Geometry: final body of the model. Coordinates: model frame, mm. Face numbers are marked on the shaded views. A direction names the side the tool comes from. Give positions to 0.01 mm unless a question says otherwise; leave off trailing zeros. Order: outer loops, then holes, each group sorted by start corner. A loop starts at its lowest first (then second) coordinate and runs counter-clockwise, first axis right, second up. Notation, with made-up numbers: (16, 37.5) -> (21, 37.5) arc R28 ccw to (21, 62.5) -> close; hole circle Ø3 at (-29.5, 46). An arc over 180 degrees is marked (long way). Answer in a Markdown table with one row per item. Add a question column.
Q1. Cut plane C-C on y = -7.5. Return the cut outline in (x, z), and give its area (3 significant figures).
Q2. Pull-direction query (Y, two-part tool) for the marked faces 1, 2, 3 and 4; classes: +Y half, -Y half, draft (parallel to the pull), parting line (faces both ways), or undercut.
Q3. Cut plane B-B on z = 5.1. Return the cut outline in (x, y), and give its area (3 significant figures).
Q4. Line query: line 1 along Z through (x, y) = (11, 20); line 2 along X through (y, z) = (-11, 4.85); line 3 along Y through (x, z) = (10, 1.75). Output: solid intervals per line, ascending. Write a range as from..to.
Q5. Cut plane A-A on x = -2.5. Return the cut outline in (y, z), and give its area (3 significant figures).
Q6. Set-up query: the marked faces 5, 6 and 7. Return all of +Z, -Z, +X, -X, +Y, -Y with unobstructed straight access to the full face (end or side cutting, diameter ignored); none if empty.
Q7. Cut plane D-D on x = -15.5. Return the cut outline in (y, z).
Q8. Contact query for flat-ended pins moving along their axis: P1, Ø2, axis at x = 14, z = 4, coming from the -Y side; P2, Ø1.8, axis at x = -10, z = 1.5, coming from the +Y side. Output: stop coordinate, or through.
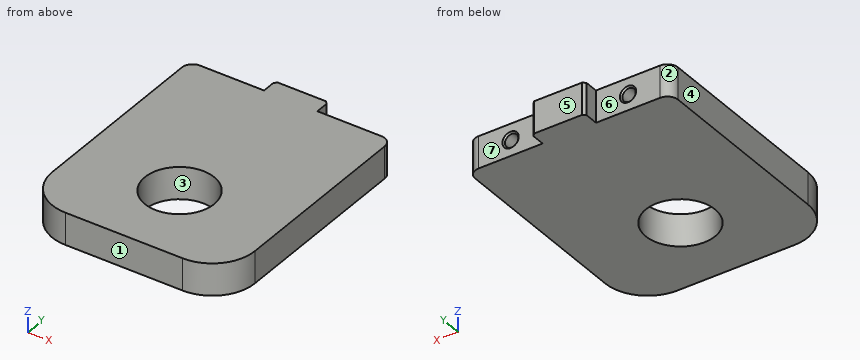
from build123d import *

# Parameters (mm, degrees)
SKETCH_1_W                   = 38
SKETCH_1_H                   = 45
EXTRUDE_1_DEPTH              = 6
SKETCH_2_R                   = 6.5
CUT_EXTRUDE_1_DEPTH          = 31.054117854
FILLET_1_R                   = 2
FILLET_2_R                   = 8
SKETCH_3_W                   = 10
SKETCH_3_H                   = 3
EXTRUDE_2_DEPTH              = 6
CHAMFER_1_SIZE               = 0.5
HOLE_WIZARD_M3_1_D           = 2.5
HOLE_WIZARD_M3_1_DEPTH       = 7.5
HOLE_WIZARD_M3_1_CSINK_D     = 3.05
HOLE_WIZARD_M3_1_CSINK_ANGLE = 90
HOLE_WIZARD_M3_1_TIP         = 0.751075774


with BuildPart() as part:
    # 草图1 → 凸台-拉伸1 (new body)
    with BuildSketch(Plane.XY):
        Rectangle(SKETCH_1_W, SKETCH_1_H)
    extrude(amount=EXTRUDE_1_DEPTH)

    # 草图2 → 切除-拉伸1 (cut, through all)
    with BuildSketch(Plane.XY.offset(6)):
        with Locations((0, -7.5)):
            Circle(SKETCH_2_R)
    extrude(amount=-CUT_EXTRUDE_1_DEPTH, mode=Mode.SUBTRACT)

    # 圆角1
    fillet_1_edges = [part.edges().sort_by_distance(p)[0] for p in [
        (-19, 22.5, 3),
        (19, 22.5, 3),
    ]]
    fillet(fillet_1_edges, radius=FILLET_1_R)

    # 圆角2
    fillet_2_edges = [part.edges().sort_by_distance(p)[0] for p in [
        (19, -22.5, 3),
        (-19, -22.5, 3),
    ]]
    fillet(fillet_2_edges, radius=FILLET_2_R)

    # 草图3 → 凸台-拉伸2 (add)
    with BuildSketch(Plane.XY.offset(6)):
        with Locations((0, 24)):
            Rectangle(SKETCH_3_W, SKETCH_3_H)
    extrude(amount=-EXTRUDE_2_DEPTH)

    # 倒角1
    chamfer_1_edges = [part.edges().sort_by_distance(p)[0] for p in [
        (-5, 25.5, 3),
        (5, 25.5, 3),
    ]]
    chamfer(chamfer_1_edges, length=CHAMFER_1_SIZE)

    # M3 螺纹孔1
    with Locations(Plane(origin=(-11, 22.5, 3), x_dir=(0, 0, 1), z_dir=(0, 1, 0))):
        with Locations((0, 0), (0, 22)):
            CounterSinkHole(HOLE_WIZARD_M3_1_D / 2, HOLE_WIZARD_M3_1_CSINK_D / 2, depth=HOLE_WIZARD_M3_1_DEPTH, counter_sink_angle=HOLE_WIZARD_M3_1_CSINK_ANGLE)
            with Locations((0, 0, -(HOLE_WIZARD_M3_1_DEPTH + HOLE_WIZARD_M3_1_TIP / 2))):  # 118° drill point
                Cone(0, HOLE_WIZARD_M3_1_D / 2, HOLE_WIZARD_M3_1_TIP, mode=Mode.SUBTRACT)


solid = part.part
Completed:
| question | item | result |
|---|---|---|
| 1 | outline | (-19, 0) -> (-6.5, 0) -> (-6.5, 6) -> (-19, 6) -> close; (6.5, 0) -> (19, 0) -> (19, 6) -> (6.5, 6) -> close |
| 1 | area | 150 mm² |
| 2 | face 1 | -Y half |
| 2 | face 2 | +Y half |
| 2 | face 3 | undercut |
| 2 | face 4 | draft |
| 3 | outline | (-19, -14.5) arc R8 ccw to (-11, -22.5) -> (11, -22.5) arc R8 ccw to (19, -14.5) -> (19, 20.5) arc R2 ccw to (17, 22.5) -> (5, 22.5) -> (5, 25) -> (4.5, 25.5) -> (-4.5, 25.5) -> (-5, 25) -> (-5, 22.5) -> (-17, 22.5) arc R2 ccw to (-19, 20.5) -> close; hole circle Ø13 at (0, -7.5) |
| 3 | area | 1,580 mm² |
| 4 | line 1 | z = 0..1.75, 4.25..6 |
| 4 | line 2 | x = -19..-5.48, 5.48..19 |
| 4 | line 3 | y = -22.5..22.5 |
| 5 | outline | (-22.5, 0) -> (-13.5, 0) -> (-13.5, 6) -> (-22.5, 6) -> close; (-1.5, 0) -> (25.5, 0) -> (25.5, 6) -> (-1.5, 6) -> close |
| 5 | area | 216 mm² |
| 6 | face 5 | +Z, -Z, +X, -X, +Y |
| 6 | face 6 | +Z, -Z, -X, +Y |
| 6 | face 7 | +Z, -Z, +X, +Y |
| 7 | outline | (-21.11, 0) -> (22.5, 0) -> (22.5, 6) -> (-21.11, 6) -> close |
| 8 | P1 | stops at y = -22.25 |
| 8 | P2 | stops at y = 22.5 |
